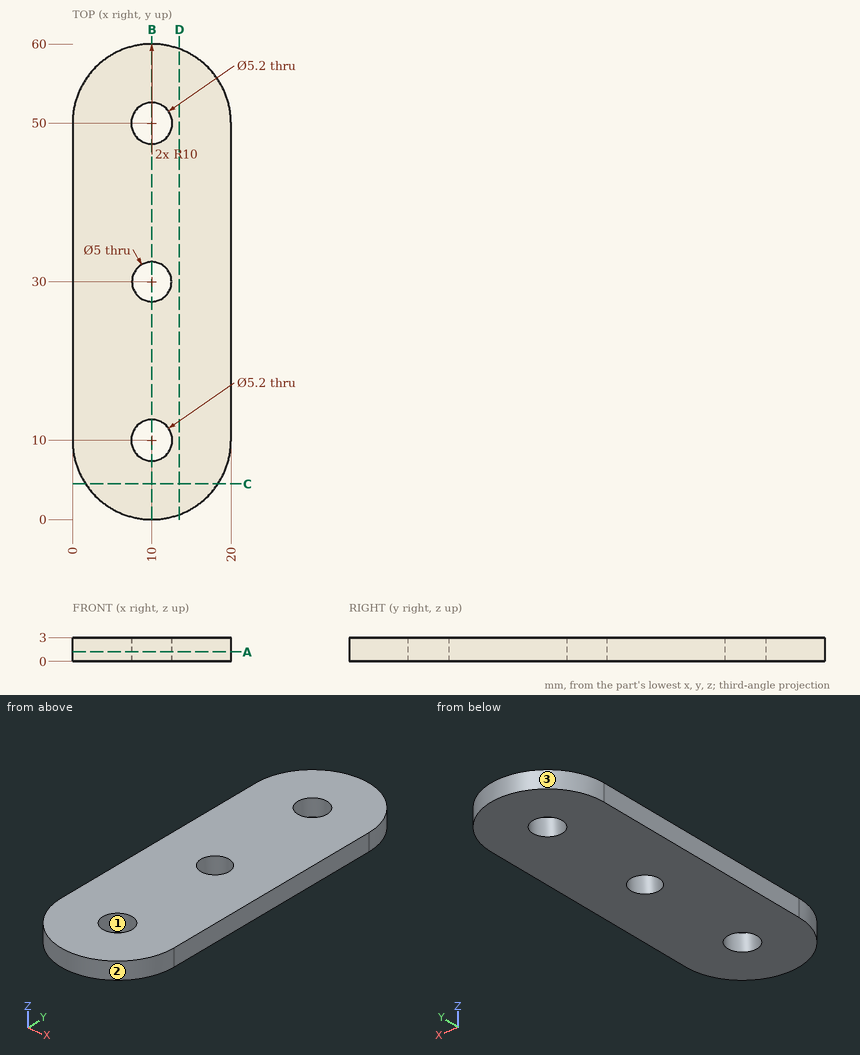
Input: dimensioned drawing with shaded views. Units: mm. Origin: part minimum x, y, z. Coordinates: 2 decimals unless noted, no trailing zeros. Loops run counter-clockwise (first coordinate to the right, second up) from the corner with the lowest first, then second, coordinate; pieces in that order, holes last. Notation, with made-up numbers: M 27.5,-36 L 32.5,-36 A20 ccw 32.5,-30 Z; hole C -12,41 d1. An arc over 180 degrees is marked long. Put each result on its own line as item: value.
(1) Draft query along Y for the marked faces 1, 2 and 3. Return one class per face: pulls with the +Y half, pulls with the -Y half, needs draft (parallel to the pull), parting line crosses it, or undercut.
Answer sheet:
face 1: undercut
face 2: pulls with the -Y half
face 3: pulls with the +Y half
(2) Cut plane C-C on y = 4.5. Return the cut outline in (x, z).
Answer sheet:
outline: M 1.65,0 L 18.35,0 L 18.35,3 L 1.65,3 Z
(3) Cut plane D-D on x = 13.5. Return the cut outline in (y, z), then the cut area to 3 significant figures.
Answer sheet:
outline: M 0.63,0 L 59.37,0 L 59.37,3 L 0.63,3 Z
area: 176 mm^2
(4) Cut plane B-B on x = 10. Return the cut outline in (y, z), then the cut area to 3 significant figures.
Answer sheet:
outline: M 0,0 L 7.4,0 L 7.4,3 L 0,3 Z; M 12.6,0 L 27.5,0 L 27.5,3 L 12.6,3 Z; M 32.5,0 L 47.4,0 L 47.4,3 L 32.5,3 Z; M 52.6,0 L 60,0 L 60,3 L 52.6,3 Z
area: 134 mm^2
(5) First-contact query: pin 1 (4.5 mm diameter, centred on x = 10, y = 10, fed in from +Z); pin 2 (1 mm diameter, centred on x = 17.5, z = 2.5, fed in from +Y); pin 3 (1 mm diameter, centred on x = 16.5, z = 1.5, fed in from +Y). Flat tips, straight axial feed; report the tip coordinate or a pass-through.
Answer sheet:
pin 1: passes through
pin 2: stops at y = 57.14
pin 3: stops at y = 58
(6) Material intervals for probe 1 along Y at (x, z) = (10, 1.95); probe 2 along Y at (x, z) = (8.25, 1.5); probe 3 along X at (y, z) = (28, 2.6), sorted ascending.
Answer sheet:
probe 1: y = 0 to 7.4, 12.6 to 27.5, 32.5 to 47.4, 52.6 to 60
probe 2: y = 0.15 to 8.08, 11.92 to 28.21, 31.79 to 48.08, 51.92 to 59.85
probe 3: x = 0 to 8.5, 11.5 to 20
(7) Cut plane A-A on z = 1.2. Return the cut outline in (x, y).
Answer sheet:
outline: M 0,10 A10 ccw 20,10 L 20,50 A10 ccw 0,50 Z; hole C 10,10 d5.2; hole C 10,50 d5.2; hole C 10,30 d5
